from build123d import *

# Parameters (mm, degrees)
SKETCH1_W                                     = 174.879
SKETCH1_H                                     = 19.05
BOSS_EXTRUDE1_DEPTH                           = 3.175
F_10_32_TAPPED_HOLE1_D                        = 4.0386
F_10_32_TAPPED_HOLE1_DEPTH                    = 11.938
F_10_32_TAPPED_HOLE1_TIP                      = 1.213317848
CSK_FOR_8_FLAT_HEAD_SOCKET_CAP_SCREW1_A_COUNT = 2
CSK_FOR_8_FLAT_HEAD_SOCKET_CAP_SCREW1_A_PITCH = 154.559


with BuildPart() as part:
    # Sketch1 → Boss-Extrude1 (new body)
    with BuildSketch(Plane(origin=(0, 0, 0), x_dir=(1, 0, 0), z_dir=(0, 1, 0))):
        Rectangle(SKETCH1_W, SKETCH1_H)
    extrude(amount=BOSS_EXTRUDE1_DEPTH)

    # #10-32 Tapped Hole1
    with Locations(Plane(origin=(0, 3.175, 0), x_dir=(-1, 0, 0), z_dir=(0, 1, 0))):
        with Locations((34.163, 0), (-34.163, 0)):
            Hole(F_10_32_TAPPED_HOLE1_D / 2, depth=F_10_32_TAPPED_HOLE1_DEPTH)
            with Locations((0, 0, -(F_10_32_TAPPED_HOLE1_DEPTH + F_10_32_TAPPED_HOLE1_TIP / 2))):  # 118° drill point
                Cone(0, F_10_32_TAPPED_HOLE1_D / 2, F_10_32_TAPPED_HOLE1_TIP, mode=Mode.SUBTRACT)

    # Sketch10 → CSK for #8 Flat Head Socket Cap Screw1 (revolve, cut)
    with BuildSketch(Plane(origin=(-77.2795, 3.175, 0), x_dir=(0, 0, 1), z_dir=(1, 0, 0))):
        Polygon((0, 0), (0, 3.175), (2.2479, 3.175), (2.2479, 2.658961536), (4.5593, 0), align=None)
    csk_for_8_flat_head_socket_cap_screw1 = revolve(axis=Axis((-77.2795, 9.525, 0), (0, -1, 0)), mode=Mode.SUBTRACT)

    # CSK for #8 Flat Head Socket Cap Screw1 a: CSK for #8 Flat Head Socket Cap Screw1 ×2
    with Locations(*[(i * CSK_FOR_8_FLAT_HEAD_SOCKET_CAP_SCREW1_A_PITCH, 0, 0) for i in range(1, CSK_FOR_8_FLAT_HEAD_SOCKET_CAP_SCREW1_A_COUNT)]):
        add(csk_for_8_flat_head_socket_cap_screw1, mode=Mode.SUBTRACT)


solid = part.part
Could you check a few things on this model? Use its own coordinates, in mm. Give positions to 0.01 mm unless a question says otherwise; leave off trailing zeros. Order: outer loops, then holes, each group sorted by start corner. A loop starts at its lowest first (then second) coordinate and runs counter-clockwise, first axis right, second up.
Item 1: If we mould it in two halves opening along X, with no side actions, what happens to faces 1 (the face through (-87.44, 2, 0)), 2 (the face through (-1, 0, 0)), 3 (the face through (36.09, 1.57, 0.61))? For each: pulls with the +X half, pulls with the -X half, needs draft (parallel to the pull), parting line crosses it, or undercut.
Item 2: If we section it at A-A, the plane z = 0: Write out the boundary of the cut face in (x, y) (1 decimal), plus the area to 3 significant figures.
Item 3: I need wall thicknesses on line 1 (Z direction, x = 34.5, y = 0.95) (3 decimals); line 2 (X direction, y = 2.5, z = 1); line 3 (X direction, y = 1.1, z = -1.25). Which ranges of each line are inside material? Lowest first, please.
Item 4: If we section it at B-B, the plane y = 1.1: Write out the boundary of the cut face in (x, z) (1 decimal).
Values:
1. face 1: pulls with the -X half
1. face 2: needs draft
1. face 3: undercut
2. outline: (-87.4, 0) - (-79.5, 0) - (-79.5, 0.5) - (-81.8, 3.2) - (-87.4, 3.2) - close; (-75, 0) - (-36.2, 0) - (-36.2, 3.2) - (-72.7, 3.2) - (-75, 0.5) - close; (-32.1, 0) - (32.1, 0) - (32.1, 3.2) - (-32.1, 3.2) - close; (36.2, 0) - (75, 0) - (75, 0.5) - (72.7, 3.2) - (36.2, 3.2) - close; (79.5, 0) - (87.4, 0) - (87.4, 3.2) - (81.8, 3.2) - (79.5, 0.5) - close
2. area: 489 mm2
3. line 1: z = -9.525 to -1.991, 1.991 to 9.525
3. line 2: x = -87.44 to -81.12, -73.43 to -35.92, -32.41 to 32.41, 35.92 to 73.43, 81.12 to 87.44
3. line 3: x = -87.44 to -79.74, -74.82 to -35.75, -32.58 to 32.58, 35.75 to 74.82, 79.74 to 87.44
4. outline: (-87.4, -9.5) - (87.4, -9.5) - (87.4, 9.5) - (-87.4, 9.5) - close; hole circle Ø5.5 at (-77.3, 0); hole circle Ø4 at (-34.2, 0); hole circle Ø4 at (34.2, 0); hole circle Ø5.5 at (77.3, 0)
